CAD build for the part. Positions are in the model's coordinates, mm. A direction names the side the tool comes from. Coordinates: 2 decimals unless noted, no trailing zeros. Loops run counter-clockwise (first coordinate to the right, second up) from the corner with the lowest first, then second, coordinate; pieces in that order, holes last.
1) Saw through at A-A, the plane x = 0. Write the cut outline in (y, z), and give its area (3 significant figures).
2) Saw through at C-C, the plane z = -6.5. Write the cut outline in (x, y).
3) Wall check: line 1 along Y through (x, z) = (0, 7.5); line 2 along X through (y, z) = (0.5, 7.5); line 3 along Z through (x, y) = (12.5, -3). Give the ranges that are in metal, low to high.
4) Two-plate mould, pull along X, no slides. Class faces 1 (the cylindrical face through (-4.01, -18.06, -46.14)), 2 (the flat face through (14, 11, 17.71)), 3 (the flat face through (0, 0, 0)): +X half, -X half, draft (parallel to the pull), parting line (faces both ways), or undercut.
5) Pin check, flat tips, straight feed: pin 1 Ø4 at (y, z) = (5.5, -46) entering from +X; pin 2 Ø12 at (y, z) = (-4.5, -21.5) entering from +X; pin 3 Ø4 at (x, z) = (1.5, 5.5) entering from +Y; pin 4 Ø6 at (x, z) = (3.5, -62.5) entering from -Y. Stop position of each tip, or through.
6) Which spindle directions (+Z, -Z, +X, -X, +Y, -Y) get a long thin tool onto all of the face, cutting with end or side? Do faces 4 (the flat face through (0, 0, -91)), 5 (the cylindrical face through (-14.6, -11.2, 8.7)). Say none if no direction does.
```python
from build123d import *

# Parameters (mm, degrees)
SKETCH1_R           = 18.4
SKETCH1_R_2         = 17.4
BOSS_EXTRUDE1_DEPTH = 17.71
BOSS_EXTRUDE2_START = -91
SKETCH1_2_R         = 18.5
SKETCH1_2_R_2       = 17.4
SKETCH1_2_R_3       = 18.4
BOSS_EXTRUDE2_DEPTH = 91


with BuildPart() as part:
    # Sketch1 → Boss-Extrude1 (new body)
    with BuildSketch(Plane.XY):
        Circle(SKETCH1_R)
        Circle(SKETCH1_R_2, mode=Mode.SUBTRACT)
    extrude(amount=BOSS_EXTRUDE1_DEPTH)

    # Sketch1<2> → Boss-Extrude2 (add)
    # profile 1 of 3: a face of its own
    with BuildSketch(Plane.XY.offset(BOSS_EXTRUDE2_START)):
        Circle(SKETCH1_2_R)
        Circle(SKETCH1_2_R_2, mode=Mode.SUBTRACT)
    # profile 2 of 3: a face of its own
    with BuildSketch(Plane.XY.offset(BOSS_EXTRUDE2_START)):
        Circle(SKETCH1_2_R)
        Circle(SKETCH1_2_R_3, mode=Mode.SUBTRACT)
    # profile 3 of 3: a face of its own
    with BuildSketch(Plane.XY.offset(BOSS_EXTRUDE2_START)):
        Circle(SKETCH1_2_R_2)
    extrude(amount=BOSS_EXTRUDE2_DEPTH)


solid = part.part
```
Data:
1. outline: (-18.5, -91) - (18.5, -91) - (18.5, 0) - (18.4, 0) - (18.4, 17.71) - (17.4, 17.71) - (17.4, 0) - (-17.4, 0) - (-17.4, 17.71) - (-18.4, 17.71) - (-18.4, 0) - (-18.5, 0) - close
1. area: 3,400 mm2
2. outline: circle Ø37 at (0, 0)
3. line 1: y = -18.4 to -17.4, 17.4 to 18.4
3. line 2: x = -18.39 to -17.39, 17.39 to 18.39
3. line 3: z = -91 to 0
4. face 1: parting line
4. face 2: draft
4. face 3: undercut
5. pin 1: stops at x = 18.17
5. pin 2: stops at x = 18.5
5. pin 3: stops at y = 18.4
5. pin 4: stops at y = -18.49
6. face 4: -Z, +X, -X, +Y, -Y
6. face 5: +Z
